Geometry check sheet. Reference: the model listing, model coordinates, mm. Coordinates: 2 decimals unless noted, no trailing zeros. Loops run counter-clockwise (first coordinate to the right, second up) from the corner with the lowest first, then second, coordinate; pieces in that order, holes last. Notation, with made-up numbers: (-20, -17) -> (15, -17) arc R21 ccw to (15, -5) -> close; hole circle Ø8 at (86, 69.25). An arc over 180 degrees is marked (long way). Answer as a JSON object with one key per item and string values.
from build123d import *

# Parameters (mm, degrees)
F0_R     = 8
F1_DEPTH = 23
F2_T     = -5.5
F3_SIZE  = 1


with BuildPart() as f1:
    # F0 (on Top) → F1 (new body)
    with BuildSketch(Plane.XY):
        Circle(F0_R)
    extrude(amount=-F1_DEPTH)

    # F2
    f2_openings = [f1.faces().sort_by_distance(p)[0] for p in [
        (0, 0, 0),
        (0, 0, -23),
    ]]
    offset(amount=F2_T, openings=f2_openings)

    # F3
    f3_edges = [f1.edges().sort_by_distance(p)[0] for p in [
        (-2.5, 0, 0),
    ]]
    chamfer(f3_edges, length=F3_SIZE)


solid = f1.part
1. Section check D-D, the plane x = -6.25. Record the boundary of the cut face in (y, z), then the cut area to 3 significant figures.
Evaluation:
{"outline": "(-4.99, -23) -> (4.99, -23) -> (4.99, 0) -> (-4.99, 0) -> close", "area": "230 mm^2"}
2. Thickness scan on probe 1 along Y at (x, z) = (0, -7.5); probe 2 along X at (y, z) = (1.75, -3). Record the ranges inside material, lowest first. Write a range as from..to.
Evaluation:
{"probe 1": "y = -8..-2.5, 2.5..8", "probe 2": "x = -7.81..-1.79, 1.79..7.81"}
3. Section check C-C, the plane z = -13.5. Record the boundary of the cut face in (x, y), then the cut area to 3 significant figures.
Evaluation:
{"outline": "circle Ø16 at (0, 0); hole circle Ø5 at (0, 0)", "area": "181 mm^2"}
4. Depth check by flat-ended pin: P1, Ø2, axis at x = -5, z = -8.5, coming from the +Y side; P2, Ø1, axis at x = -4, z = -14, coming from the +Y side; P3, Ø8, axis at y = -5.5, z = -3.5, coming from the -X side. Enter the tip coordinate at first touch or a pass-through.
Evaluation:
{"P1": "stops at y = 6.93", "P2": "stops at y = 7.19", "P3": "stops at x = -7.86"}
5. Mould release check, pull along Y, two halves, no side actions. Record for faces 1 (the face through (3.4, -1.7, 0)), 2 (the face through (-0.54, -2.44, -11.85)), 3 (the face through (-1.73, -7.81, -11.34)): released by +Y, released by -Y, zero draft, split by the parting line, or undercut.
Evaluation:
{"face 1": "zero draft", "face 2": "undercut", "face 3": "split by the parting line"}
6. Section check A-A, the plane x = 0. Record the boundary of the cut face in (y, z), then the cut area to 3 significant figures.
Evaluation:
{"outline": "(-8, -23) -> (-2.5, -23) -> (-2.5, -1) -> (-3.5, 0) -> (-8, 0) -> close; (2.5, -23) -> (8, -23) -> (8, 0) -> (3.5, 0) -> (2.5, -1) -> close", "area": "252 mm^2"}
